Could you check a few things on this drawing? It's one solid part, dimensions in mm from its lowest x, y, z. A direction names the side the tool comes from. Give positions to 0.01 mm unless a question says otherwise; leave off trailing zeros. Write each loop counter-clockwise with the first axis right and the second up, starting at its lowest first coordinate (ties: lowest second). Pieces come first, ordered by that corner, then holes. Notation, with made-up numbers: M 54.5,33.25 L 58.5,33.25 A19 ccw 58.5,46.25 Z; hole C -33.75,4 d6. An arc over 180 degrees is marked long. Write each question's results on one line, items separated by ' | '. Start each with the question number.
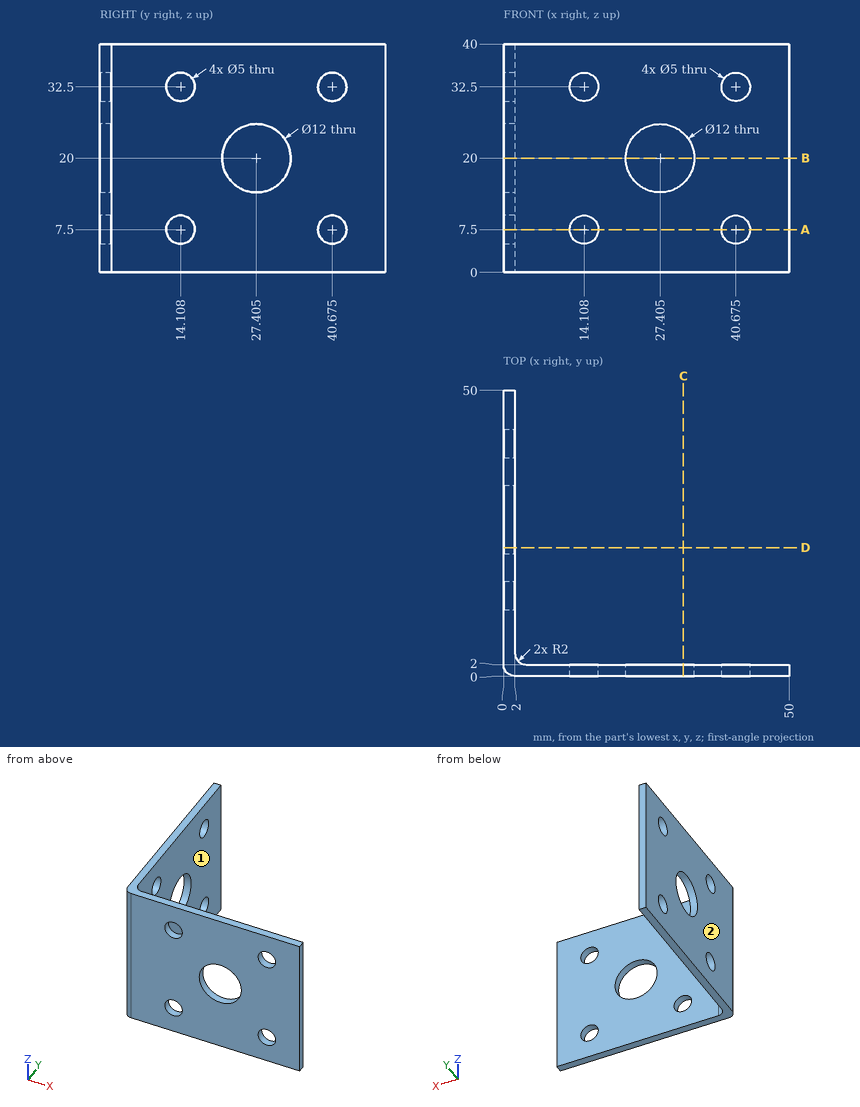
Q1. If we section it at C-C (x = 31.5): Please give me the cut outline in (y, z) (1 decimal).
Q2. If we section it at B-B (z = 20): Please give me the cut outline in (x, y) (1 decimal), plus the area to 3 significant figures.
Q3. For the marked faces 1 and 2, which set-ups out of +Z, -Z, +X, -X, +Y, -Y let a thin tool reach every point of the face, with its end or its side?
Q4. If we section it at A-A (z = 7.5): Please give me the cut outline in (x, y) (1 decimal).
Q5. If we section it at D-D (y = 22.5): Please give me the cut outline in (x, z) (1 decimal).
Q6. I'm going to push flat-ended pins straight in: P1, Ø3, axis at x = 14.11, z = 32.5, coming from the -Y side; P2, Ø6.5, axis at y = 40.68, z = 32.5, coming from the +X side; P3, Ø20, axis at x = 37.5, z = 26.5, coming from the +Y side. Where does each tip first touch, or does it pass through?
Q7. Please list where these lines run through material, in increasing order: line 1 (Y direction, x = 1.5, z = 32.5) (1 decimal); line 2 (X direction, y = 34.5, z = 17). Write a range as [from, to].
Determined:
1) outline: M 0,0 L 2,0 L 2,15.6 L 0,15.6 Z; M 0,24.4 L 2,24.4 L 2,40 L 0,40 Z
2) outline: M 0,2 A2 ccw 2,0 L 21.4,0 L 21.4,2 L 4,2 A2 cw 2,4 L 2,21.4 L 0,21.4 Z; M 0,33.4 L 2,33.4 L 2,50 L 0,50 Z; M 33.4,0 L 50,0 L 50,2 L 33.4,2 Z | area: 148 mm²
3) face 1: +Z, -Z, +X, +Y | face 2: +Z, -Z, -X, +Y, -Y
4) outline: M 0,2 A2 ccw 2,0 L 11.6,0 L 11.6,2 L 4,2 A2 cw 2,4 L 2,11.6 L 0,11.6 Z; M 0,16.6 L 2,16.6 L 2,38.2 L 0,38.2 Z; M 0,43.2 L 2,43.2 L 2,50 L 0,50 Z; M 16.6,0 L 38.2,0 L 38.2,2 L 16.6,2 Z; M 43.2,0 L 50,0 L 50,2 L 43.2,2 Z
5) outline: M 0,0 L 2,0 L 2,16.5 L 0,16.5 Z; M 0,23.5 L 2,23.5 L 2,40 L 0,40 Z
6) P1: passes through | P2: stops at x = 2 | P3: stops at y = 2
7) line 1: y = [0.1, 11.6], [16.6, 38.2], [43.2, 50] | line 2: x = [0, 2]
